Check sheet for the modelled part. Datum: model origin and axes. Units: mm. A direction names the side the tool comes from. Give positions to 0.01 mm unless a question says otherwise; leave off trailing zeros. Write each loop counter-clockwise with the first axis right and the second up, starting at its lowest first coordinate (ties: lowest second). Pieces come first, ordered by that corner, then holes. Notation, with made-up numbers: (51.25, -29.5) -> (79.25, -29.5) arc R17 cw to (79.25, -10.5) -> close; hole circle Ø9 at (-39.5, 34.25). An arc over 180 degrees is marked (long way). Answer as a JSON object with one key per item and string values.
from build123d import *

# Parameters (mm, degrees)
SKETCH1_R           = 2
BOSS_EXTRUDE1_DEPTH = 4


with BuildPart() as part:
    # Sketch1 → Boss-Extrude1 (new body)
    with BuildSketch(Plane.XY):
        Polygon((28.783278196, 114.493956315), (64.138617256, 79.138617256), (25, 40), (25, -10), (-25, -10), (-25, 40), (-25, 60.710678119), align=None)
        with Locations((-12.5, 27.5)):
            Circle(SKETCH1_R, mode=Mode.SUBTRACT)
        with Locations((12.5, 27.5)):
            Circle(SKETCH1_R, mode=Mode.SUBTRACT)
        with Locations((12.5, 2.5)):
            Circle(SKETCH1_R, mode=Mode.SUBTRACT)
        with Locations((-12.5, 2.5)):
            Circle(SKETCH1_R, mode=Mode.SUBTRACT)
        with BuildLine():
            Line((48.228714679, 84.441918115), (30.551045149, 102.119587644))
            ThreePointArc((30.551045149, 102.119587644), (27.015511244, 102.119587644), (27.015511244, 98.584053738))
            Line((27.015511244, 98.584053738), (44.693180773, 80.906384209))
            ThreePointArc((44.693180773, 80.906384209), (48.228714679, 80.906384209), (48.228714679, 84.441918115))
        make_face(mode=Mode.SUBTRACT)
    extrude(amount=BOSS_EXTRUDE1_DEPTH)


solid = part.part
1. Scan lines: L1, parallel to X at y = 39, z = 2.25; L2, parallel to X at y = 94.5, z = 3.6; L3, parallel to Y at x = 12.5, z = 2.4. Record each from-to range of solid material in increasing order. Write a range as [from, to].
Determined:
{"L1": "[-25, 25]", "L2": "[8.79, 31.1], [38.17, 48.78]", "L3": "[-10, 0.5], [4.5, 25.5], [29.5, 98.21]"}
2. Sectioned sample at C-C, the plane x = -12.5. Enter the section's corners in (y, z).
Determined:
{"outline": "(-10, 0) -> (0.5, 0) -> (0.5, 4) -> (-10, 4) -> close; (4.5, 0) -> (25.5, 0) -> (25.5, 4) -> (4.5, 4) -> close; (29.5, 0) -> (73.21, 0) -> (73.21, 4) -> (29.5, 4) -> close"}
3. Sectioned sample at A-A, the plane y = 2.5. Enter the section's corners in (x, z).
Determined:
{"outline": "(-25, 0) -> (-14.5, 0) -> (-14.5, 4) -> (-25, 4) -> close; (-10.5, 0) -> (10.5, 0) -> (10.5, 4) -> (-10.5, 4) -> close; (14.5, 0) -> (25, 0) -> (25, 4) -> (14.5, 4) -> close"}
4. Sectioned sample at B-B, the plane z = 1.45. Enter the section's corners in (x, y).
Determined:
{"outline": "(-25, -10) -> (25, -10) -> (25, 40) -> (64.14, 79.14) -> (28.78, 114.49) -> (-25, 60.71) -> close; hole circle Ø4 at (-12.5, 2.5); hole circle Ø4 at (-12.5, 27.5); hole circle Ø4 at (12.5, 2.5); hole circle Ø4 at (12.5, 27.5); hole (27.02, 98.58) -> (44.69, 80.91) arc R2.5 ccw to (48.23, 84.44) -> (30.55, 102.12) arc R2.5 ccw to start"}
5. Sectioned sample at D-D, the plane y = 92. Enter the section's corners in (x, z).
Determined:
{"outline": "(6.29, 0) -> (33.6, 0) -> (33.6, 4) -> (6.29, 4) -> close; (40.67, 0) -> (51.28, 0) -> (51.28, 4) -> (40.67, 4) -> close"}
6. Go/stop test with flat-tipped pins: P1, Ø2, axis at y = 9, z = 1.5, coming from the +X side; P2, Ø1, axis at y = 74, z = 1.5, coming from the +X side; P3, Ø3, axis at x = 12.5, y = 2.5, coming from the -Z side. Record where each tip stops, or that it passes through.
Determined:
{"P1": "x = 25", "P2": "x = 59.5", "P3": "through"}
7. Mould release check, pull along Y, two halves, no side actions. Record for faces 1 (the face through (45, 60, 2)), 2 (the face through (46.213, 97.064, 1.972)), 3 (the face through (-12.934, 25.548, 1.972)): released by +Y, released by -Y, zero draft, split by the parting line, or undercut.
Determined:
{"face 1": "released by -Y", "face 2": "released by +Y", "face 3": "undercut"}
8. Access from +Z, -Z, +X, -X, +Y, -Y to the whole of each face (thin tool, end or side, straight path). Record for faces 4 (the face through (35.7, 89.9, 2)), 5 (the face through (0, -10, 2)), 6 (the face through (25, 15, 2)).
Determined:
{"face 4": "+Z, -Z", "face 5": "+Z, -Z, +X, -X, -Y", "face 6": "+Z, -Z, +X, -Y"}
